For this review, take the finished solid that the model builds, in its own axes (mm). Coordinates: 2 decimals unless noted, no trailing zeros. Loops run counter-clockwise (first coordinate to the right, second up) from the corner with the lowest first, then second, coordinate; pieces in that order, holes last. Notation, with made-up numbers: (7.25, 5.25) -> (60.25, 5.25) arc R20 ccw to (60.25, 42.25) -> close; hole circle Ø1 at (60.5, 50.25). An arc over 180 degrees is marked (long way). One line per item, written item: value.
from build123d import *

# Parameters (mm, degrees)
SKETCH1_W           = 341.884
SKETCH1_H           = 341.884
BOSS_EXTRUDE1_DEPTH = 1.89738
SKETCH2_R           = 21.209
CUT_EXTRUDE1_DEPTH  = 2.89738
FILLET2_R           = 12.7
CUT_EXTRUDE3_DEPTH  = 2.89738
FILLET3_R           = 0.762


with BuildPart() as part:
    # Sketch1 → Boss-Extrude1 (new body)
    with BuildSketch(Plane(origin=(0, 0, 0), x_dir=(1, 0, 0), z_dir=(0, 1, 0))):
        Rectangle(SKETCH1_W, SKETCH1_H)
    extrude(amount=BOSS_EXTRUDE1_DEPTH)

    # Sketch2 → Cut-Extrude1 (cut, through all)
    with BuildSketch(Plane(origin=(0, 1.89738, 0), x_dir=(1, 0, 0), z_dir=(0, 1, 0))):
        with Locations((-139.192, -139.192)):
            Circle(SKETCH2_R)
        with Locations((-139.192, 139.192)):
            Circle(SKETCH2_R)
        with Locations((139.192, 139.192)):
            Circle(SKETCH2_R)
        with Locations((139.192, -139.192)):
            Circle(SKETCH2_R)
    extrude(amount=-CUT_EXTRUDE1_DEPTH, mode=Mode.SUBTRACT)

    # Fillet2
    fillet2_edges = [part.edges().sort_by_distance(p)[0] for p in [
        (-170.942, 0.94869, -170.942),
        (170.942, 0.94869, -170.942),
        (170.942, 0.94869, 170.942),
        (-170.942, 0.94869, 170.942),
    ]]
    fillet(fillet2_edges, radius=FILLET2_R)

    # Sketch6 → Cut-Extrude3 (cut, through all)
    with BuildSketch(Plane(origin=(0, 1.89738, 0), x_dir=(1, 0, 0), z_dir=(0, 1, 0))):
        with BuildLine():
            Line((6.977594198, 21.916760235), (-1.287294389, 3.353516536))
            Line((-1.287294389, 3.353516536), (-19.850538088, 11.618405123))
            ThreePointArc((-19.850538088, 11.618405123), (-23.204054624, 10.331110734), (-21.916760235, 6.977594198))
            Line((-21.916760235, 6.977594198), (-3.353516536, -1.287294389))
            Line((-3.353516536, -1.287294389), (-11.618405123, -19.850538088))
            ThreePointArc((-11.618405123, -19.850538088), (-10.331110734, -23.204054624), (-6.977594198, -21.916760235))
            Line((-6.977594198, -21.916760235), (1.287294389, -3.353516536))
            Line((1.287294389, -3.353516536), (19.850538088, -11.618405123))
            ThreePointArc((19.850538088, -11.618405123), (23.204054624, -10.331110734), (21.916760235, -6.977594198))
            Line((21.916760235, -6.977594198), (3.353516536, 1.287294389))
            Line((3.353516536, 1.287294389), (11.618405123, 19.850538088))
            ThreePointArc((11.618405123, 19.850538088), (10.331110734, 23.204054624), (6.977594198, 21.916760235))
        make_face()
        with BuildLine():
            Line((-170.942, 78.193564035), (-163.205950308, 74.749252801))
            ThreePointArc((-163.205950308, 74.749252801), (-162.240479516, 72.234115399), (-164.755616918, 71.268644607))
            Line((-164.755616918, 71.268644607), (-170.942, 74.022999813))
            Line((-170.942, 74.022999813), (-170.942, 78.193564035))
        make_face()
        with BuildLine():
            Line((74.022999813, 170.942), (78.193564035, 170.942))
            Line((78.193564035, 170.942), (74.749252801, 163.205950308))
            ThreePointArc((74.749252801, 163.205950308), (72.234115399, 162.240479516), (71.268644607, 164.755616918))
            Line((71.268644607, 164.755616918), (74.022999813, 170.942))
        make_face()
        with BuildLine():
            Line((170.942, -74.022999813), (170.942, -78.193564035))
            Line((170.942, -78.193564035), (163.205950308, -74.749252801))
            ThreePointArc((163.205950308, -74.749252801), (162.240479516, -72.234115399), (164.755616918, -71.268644607))
            Line((164.755616918, -71.268644607), (170.942, -74.022999813))
        make_face()
        with BuildLine():
            Line((-74.022999813, -170.942), (-78.193564035, -170.942))
            Line((-78.193564035, -170.942), (-74.749252801, -163.205950308))
            ThreePointArc((-74.749252801, -163.205950308), (-72.234115399, -162.240479516), (-71.268644607, -164.755616918))
            Line((-71.268644607, -164.755616918), (-74.022999813, -170.942))
        make_face()
    extrude(amount=-CUT_EXTRUDE3_DEPTH, mode=Mode.SUBTRACT)

    # Fillet3
    fillet3_edges = [part.edges().sort_by_distance(p)[0] for p in [
        (78.193564035, 0.94869, -170.942),
        (74.022999813, 0.94869, -170.942),
        (-170.942, 0.94869, -74.022999813),
        (-170.942, 0.94869, -78.193564035),
        (3.353516536, 0.94869, -1.287294389),
        (1.287294389, 0.94869, 3.353516536),
        (-3.353516536, 0.94869, 1.287294389),
        (-1.287294389, 0.94869, -3.353516536),
        (-78.193564035, 0.94869, 170.942),
        (-74.022999813, 0.94869, 170.942),
        (170.942, 0.94869, 78.193564035),
        (170.942, 0.94869, 74.022999813),
    ]]
    fillet(fillet3_edges, radius=FILLET3_R)


solid = part.part
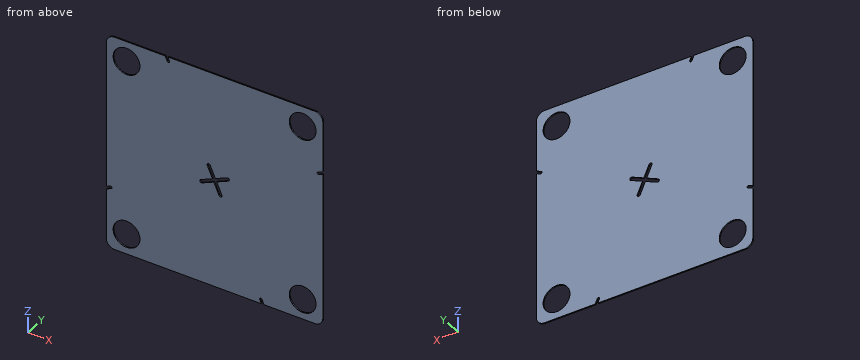
1. Take a section at B-B, the plane x = 147. Give the boundary of the cut face in (y, z).
Return value:
outline: (0, -170.94) -> (1.9, -170.94) -> (1.9, -158.91) -> (0, -158.91) -> close; (0, -119.47) -> (1.9, -119.47) -> (1.9, 119.47) -> (0, 119.47) -> close; (0, 158.91) -> (1.9, 158.91) -> (1.9, 170.94) -> (0, 170.94) -> close
2. To check wall thickness, follow probe 1 along X at (y, z) = (1.05, 121.5); probe 2 along X at (y, z) = (0.35, 11.5); probe 3 along Z at (x, y) = (134.5, 0.55). State the ranges of each line that lie inside material, in increasing order. Write a range as from..to.
Return value:
probe 1: x = -170.94..-150.89, -127.5..127.5, 150.89..170.94
probe 2: x = -170.94..-7.9, -2.34..19.58, 22.15..170.94
probe 3: z = -170.94..-159.88, -118.51..118.51, 159.88..170.94
3. Take a section at C-C, the plane y = 0.8. Give the number of separate pieces and of enclosed holes in the cut face, and give its area (3 significant figures).
Return value:
separate pieces: 1
enclosed holes: 5
area: 110,000 mm2
4. Take a section at A-A, the plane x = -133. Give the boundary of the cut face in (y, z), and give its area (3 significant figures).
Return value:
outline: (0, -170.94) -> (1.9, -170.94) -> (1.9, -159.48) -> (0, -159.48) -> close; (0, -118.91) -> (1.9, -118.91) -> (1.9, 118.91) -> (0, 118.91) -> close; (0, 159.48) -> (1.9, 159.48) -> (1.9, 170.94) -> (0, 170.94) -> close
area: 495 mm2
